Autodesk Inventor part; units mm, degrees
ref_plane "YZ Plane" through (0, 0, 0) normal (1, 0, 0) x (0, 1, 0)
ref_plane "XZ Plane" through (0, 0, 0) normal (0, 1, 0) x (-1, 0, 0)
ref_plane "XY Plane" through (0, 0, 0) normal (0, 0, 1) x (1, 0, 0)
sketch "스케치1" plane through (0, 0, 0) normal (0, 0, 1) x (1, 0, 0)
  line L0 (13.6602, -9.1135) -> (-13.6602, -9.1135)
  line L1 (-13.6602, -9.1135) -> (-13.6602, 9.1135)
  line L2 (-13.6602, 9.1135) -> (13.6602, 9.1135)
  line L3 (13.6602, 9.1135) -> (13.6602, -9.1135)
  line L4 (13.6602, -9.1135) -> (-13.6602, 9.1135) construction
  line L5 (-13.6602, -9.1135) -> (13.6602, 9.1135) construction
  point P0 (0, 0)
extrude "돌출1" add sketch "스케치1" along normal blind 20
sketch "스케치2" plane through (-13.6602, 9.1135, 0) normal (0, 1, 0) x (1, 0, 0)
  line L0 (0, -20) -> (27.3204, -20)
  line L1 (27.3204, 0) -> (27.3204, -20)
  line L2 (17.7495, -20) -> (27.3204, -20)
  line L3 (27.3204, -20) -> (27.3204, -10)
  line L4 (27.3204, -10) -> (17.7495, -10)
  line L5 (17.7495, -10) -> (17.7495, -20)
  point P0 (13.6602, 0)
extrude "돌출2" cut sketch "스케치2" against normal blind 20
sketch "스케치3" plane through (-13.6602, 9.1135, 0) normal (0, 1, 0) x (1, 0, 0)
  point P0 (13.6602, 0)
sketch "스케치4" plane through (-13.6602, 9.1135, 0) normal (0, 1, 0) x (1, 0, 0)
  line L0 (0, -20) -> (17.7495, -20)
  line L1 (6.0281, -20) -> (6.0281, 0)
  line L2 (27.3204, 0) -> (0, 0)
  line L3 (22.0453, 0) -> (22.0453, -10)
  line L4 (17.7495, -10) -> (27.3204, -10)
  line L5 (17.7495, -20) -> (17.7495, -10)
  line L6 (17.7495, -10) -> (17.7495, -20)
  line L7 (17.7495, -20) -> (6.0281, -20)
  point P0 (13.6602, 0)
extrude "돌출3" cut sketch "스케치4" against normal blind 9
sketch "스케치5" plane through (-13.6602, 0.1135, 0) normal (0, 1, 0) x (1, 0, 0)
  circle A0 centre (20.026, -4.8257) radius 1.5639
  circle A1 centre (11.6067, -15.0931) radius 2.4307
  point P0 (13.6602, 0)
extrude "돌출4" cut sketch "스케치5" against normal blind 10
fillet "모깎기1" radius 5 1 edges at (-10.6462, 9.1135, 20)
fillet "모깎기2" radius 5 1 edges at (-10.6462, 9.1135, 0)
properties part number "240503_3Dsketch11"
For this review, take the finished solid that the model builds, in its own axes (mm). A direction names the side the tool comes from. Coordinates: 2 decimals unless noted, no trailing zeros. Order: outer loops, then holes, each group sorted by start corner. A loop starts at its lowest first (then second) coordinate and runs counter-clockwise, first axis right, second up. Notation, with made-up numbers: (46, -13) -> (99, -13) arc R27 cw to (99, 13) -> close; hole circle Ø2 at (13.25, 0.5). An arc over 180 degrees is marked (long way). Answer as CSV lines item,"result".
Q1. We need section A-A (y = 1.75). State the section outline as (x, z) points, plus the area to 3 significant figures.
Model answer:
outline,"(-13.66, 0) -> (-7.63, 0) -> (-7.63, 20) -> (-13.66, 20) -> close; (8.39, 0) -> (13.66, 0) -> (13.66, 10) -> (8.39, 10) -> close"
area,"173 mm2"
Q2. We need section B-B (y = -6.5). State the section outline as (x, z) points.
Model answer:
outline,"(-13.66, 0) -> (13.66, 0) -> (13.66, 10) -> (4.09, 10) -> (4.09, 20) -> (-13.66, 20) -> close; hole circle Ø4.86 at (-2.05, 15.09); hole circle Ø3.13 at (6.37, 4.83)"
Q3. We need section C-C (z = 11). State the section outline as (x, y) points, plus the area to 3 significant figures.
Model answer:
outline,"(-13.66, -9.11) -> (4.09, -9.11) -> (4.09, 0.11) -> (-7.63, 0.11) -> (-7.63, 9.11) -> (-13.66, 9.11) -> close"
area,"218 mm2"
Q4. For faces 1 (the face through (-10.604, 7.61, 1.426)), 2 (the face through (-7.632, 5, 10)), 3 (the face through (10, -2, 10)), 4 (the face through (13.66, 0, 5)), list the 3-axis set-ups (+Z, -Z, +X, -X, +Y, -Y) from which the entire face can be reached by the end or side of a thin tool; tool diameter is ignored.
Model answer:
face 1,"-Z, -X, +Y"
face 2,"+Z, -Z, +Y"
face 3,"+Z, +X, +Y, -Y"
face 4,"+Z, -Z, +X, +Y, -Y"
Q5. We need section D-D (x = 7.25). State the section outline as (y, z) points, plus the area to 3 significant figures.
Model answer:
outline,"(-9.11, 0) -> (0.11, 0) -> (0.11, 3.54) -> (-9.11, 3.54) -> close; (-9.11, 6.12) -> (0.11, 6.12) -> (0.11, 10) -> (-9.11, 10) -> close"
area,"68.5 mm2"
Q6. Clearance check with flat-ended pins moving along their axes: pin 1 Ø2.5 at (y, z) = (6.5, 11.5) entering from +X; pin 2 Ø7.5 at (x, y) = (10, 0) entering from +Z; pin 3 Ø6 at (x, z) = (6, 7.5) entering from +Y; pin 4 Ø1.5 at (y, z) = (-3, 15.5) entering from +X. State where each tip first meets the part, or that it passes through.
Model answer:
pin 1,"stops at x = -7.63"
pin 2,"stops at z = 10"
pin 3,"stops at y = 9.11"
pin 4,"stops at x = 4.09"
Q7. Wall thickness on line 1 along X through (y, z) = (3.5, 7.25); line 2 along X through (y, z) = (-8, 17.25); line 3 along Z through (x, y) = (12.25, 0.75): over which ranges is each line inside the solid? List them lowest first. Write a range as [from, to].
Model answer:
line 1,"x = [-13.66, -7.63], [8.39, 13.66]"
line 2,"x = [-13.66, -3.17], [-0.93, 4.09]"
line 3,"z = [0, 10]"
Q8. Draft analysis for pull direction X (two halves, no side actions). For faces 5 (the face through (0, 0.114, 10)), 6 (the face through (-3, -9.114, 8)), 7 (the face through (4.089, -4, 15)), state which applies: released by +X, released by -X, zero draft, split by the parting line, or undercut.
Model answer:
face 5,"undercut"
face 6,"zero draft"
face 7,"released by +X"
